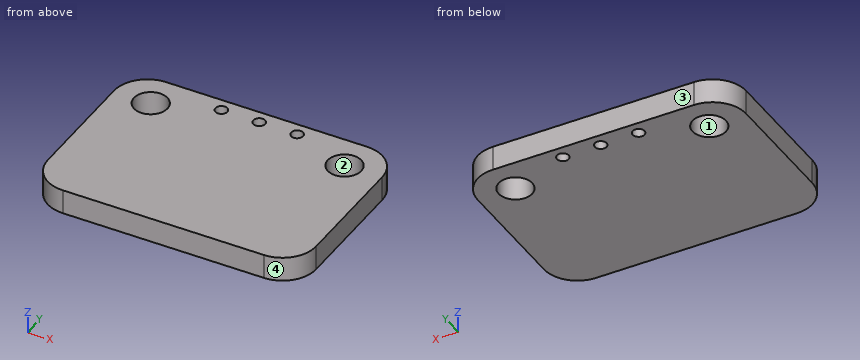
from build123d import *

# Parameters (mm, degrees)
PAD012_DEPTH    = 1.65
SKETCH037_R     = 1.125
POCKET011_DEPTH = 1.651
SKETCH038_R     = 0.4
POCKET001_DEPTH = 1.651


with BuildPart() as part:
    # Sketch036 → Pad012 (new body)
    with BuildSketch(Plane.XY):
        with BuildLine():
            Line((-6.75, 12.5), (6.75, 12.5))
            ThreePointArc((9, 10.25), (8.34099, 11.84099), (6.75, 12.5))
            Line((9, 10.25), (9, 2.25))
            ThreePointArc((6.75, 0), (8.34099, 0.65901), (9, 2.25))
            Line((6.75, 0), (-6.75, 0))
            ThreePointArc((-9, 2.25), (-8.34099, 0.65901), (-6.75, 0))
            Line((-9, 2.25), (-9, 10.25))
            ThreePointArc((-6.75, 12.5), (-8.34099, 11.84099), (-9, 10.25))
        make_face()
    extrude(amount=-PAD012_DEPTH)

    # Sketch037 → Pocket011 (cut, through all)
    with BuildSketch(Plane.XY):
        with Locations((-6.5, 10.2)):
            Circle(SKETCH037_R)
        with Locations((6.5, 10.2)):
            Circle(SKETCH037_R)
    extrude(amount=-POCKET011_DEPTH, mode=Mode.SUBTRACT)

    # Sketch038 → Pocket001 (cut, through all)
    with BuildSketch(Plane.XY):
        with Locations((0, 11.61)):
            Circle(SKETCH038_R)
        with Locations((2.54, 11.61)):
            Circle(SKETCH038_R)
        with Locations((-2.54, 11.61)):
            Circle(SKETCH038_R)
    extrude(amount=-POCKET001_DEPTH, mode=Mode.SUBTRACT)


solid = part.part
Read the model definition and answer for the solid it produces. Units are mm, in the model's axes. Face numbers are marked on the shaded views. Coordinates: 2 decimals unless noted, no trailing zeros. Loops run counter-clockwise (first coordinate to the right, second up) from the corner with the lowest first, then second, coordinate; pieces in that order, holes last. Notation, with made-up numbers: (75, 36) - (109, 36) arc R21 ccw to (109, 53) - close; hole circle Ø10 at (22, 28.5). An arc over 180 degrees is marked (long way). Answer in a Markdown table with one row per item.
Q1. Find section A-A on x = 6.5. Write down the section's boundary in (y, z) (3 decimals), plus the area to 3 significant figures.
Here are the results:
| item | result |
|---|---|
| outline | (0, -1.65) - (9.075, -1.65) - (9.075, 0) - (0, 0) - close; (11.325, -1.65) - (12.5, -1.65) - (12.5, 0) - (11.325, 0) - close |
| area | 16.9 mm^2 |
Q2. Find section B-B on z = -0.4. Write down the section's boundary in (x, y) (3 decimals).
Here are the results:
| item | result |
|---|---|
| outline | (-9, 2.25) arc R2.25 ccw to (-6.75, 0) - (6.75, 0) arc R2.25 ccw to (9, 2.25) - (9, 10.25) arc R2.25 ccw to (6.75, 12.5) - (-6.75, 12.5) arc R2.25 ccw to (-9, 10.25) - close; hole circle Ø2.25 at (-6.5, 10.2); hole circle Ø0.8 at (-2.54, 11.61); hole circle Ø0.8 at (0, 11.61); hole circle Ø0.8 at (2.54, 11.61); hole circle Ø2.25 at (6.5, 10.2) |
Q3. Find section C-C on y = 11.61. Write down the section's boundary in (x, z), plus the area to 3 significant figures.
Here are the results:
| item | result |
|---|---|
| outline | (-8.54, -1.65) - (-2.94, -1.65) - (-2.94, 0) - (-8.54, 0) - close; (-2.14, -1.65) - (-0.4, -1.65) - (-0.4, 0) - (-2.14, 0) - close; (0.4, -1.65) - (2.14, -1.65) - (2.14, 0) - (0.4, 0) - close; (2.94, -1.65) - (8.54, -1.65) - (8.54, 0) - (2.94, 0) - close |
| area | 24.2 mm^2 |
Q4. Find section D-D on x = 0. Write down the section's boundary in (y, z), plus the area to 3 significant figures.
Here are the results:
| item | result |
|---|---|
| outline | (0, -1.65) - (11.21, -1.65) - (11.21, 0) - (0, 0) - close; (12.01, -1.65) - (12.5, -1.65) - (12.5, 0) - (12.01, 0) - close |
| area | 19.3 mm^2 |
Q5. Straight lines are drawn through the part: line 1 along Y through (x, z) = (-6.5, -0.9) (3 decimals); line 2 along X through (y, z) = (9.5, -0.85); line 3 along X through (y, z) = (11.5, -0.25). For each, find the intervals that lie inside material, in ascending order. Write a range as [from, to].
Here are the results:
| item | result |
|---|---|
| line 1 | y = [0, 9.075], [11.325, 12.5] |
| line 2 | x = [-9, -7.38], [-5.62, 5.62], [7.38, 9] |
| line 3 | x = [-8.62, -2.92], [-2.16, -0.38], [0.38, 2.16], [2.92, 8.62] |
Q6. The mould has two halves that part along X. Classify the marked faces 1, 2, 3 and 4: pulls with the +X half, pulls with the -X half, needs draft (parallel to the pull), parting line crosses it, or undercut.
Here are the results:
| item | result |
|---|---|
| face 1 | undercut |
| face 2 | undercut |
| face 3 | needs draft |
| face 4 | pulls with the +X half |
